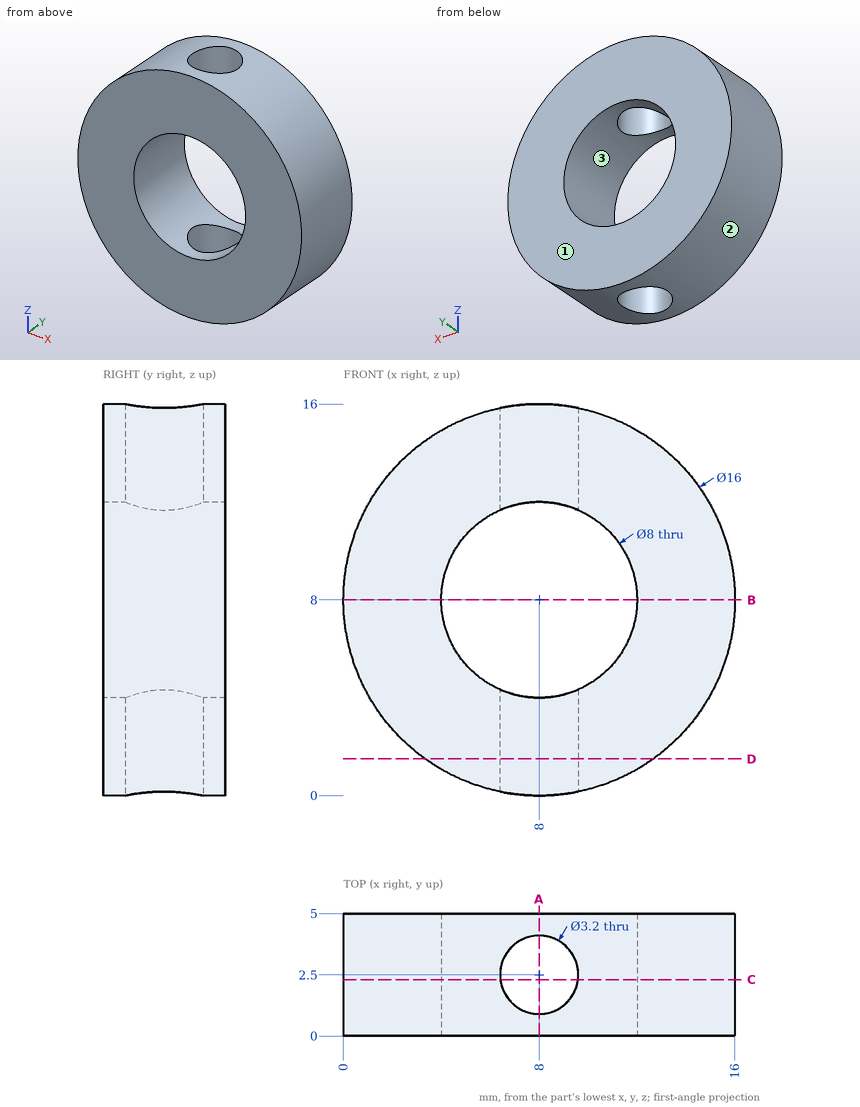
Can you work these out from the drawing? Everything is in mm from the part's minimum corner. Coordinates: 2 decimals unless noted, no trailing zeros. Loops run counter-clockwise (first coordinate to the right, second up) from the corner with the lowest first, then second, coordinate; pieces in that order, holes last. Notation, with made-up numbers: M -30,20.25 L 5,20.25 A6 ccw 5,29.25 Z; hole C 23,-14 d8. An arc over 180 degrees is marked long. Put each result on its own line as item: value. Start each with the question number.
(1) Suppose I cut it at D-D on z = 1.5. Please give me the cut outline in (x, y), then the cut area to 3 significant figures.
(2) Thinking about a two-plate mould opening in Z: for the marked faces 1, 2 and 3, which applies, pulls with the +Z half, pulls with the -Z half, needs draft (parallel to the pull), parting line crosses it, or undercut?
(3) Will this pin go through, and if not, where does the flat tip stop? P1, Ø1, axis at y = 1, z = 5, coming from the -X side.
(4) Suppose I cut it at C-C on y = 2.3. Please give me the cut outline in (x, z).
(5) Suppose I cut it at A-A on x = 8. Please give me the cut outline in (y, z), then the cut area to 3 significant figures.
(6) Suppose I cut it at B-B on z = 8. Please give me the cut outline in (x, y).
(7) I need wall thicknesses on line 1 (X direction, y = 2.35, z = 8.5); line 2 (Z direction, x = 4.5, y = 0.4); line 3 (X direction, y = 3.75, z = 14.5). Which ranges of each line are inside material? Lowest first, please. Write a range as from..to.
Solutions:
1. outline: M 3.34,0 L 12.66,0 L 12.66,5 L 3.34,5 Z; hole C 8,2.5 d3.2
1. area: 38.6 mm2
2. face 1: needs draft
2. face 2: parting line crosses it
2. face 3: undercut
3. P1: stops at x = 0.4
4. outline: M 6.41,0.16 L 6.41,4.33 A4 cw 6.41,11.67 L 6.41,15.84 A8 ccw Z; M 9.59,0.16 A8 ccw 9.59,15.84 L 9.59,11.67 A4 cw 9.59,4.33 Z
5. outline: M 0,0 L 0.9,0 L 0.9,4 L 0,4 Z; M 0,12 L 0.9,12 L 0.9,16 L 0,16 Z; M 4.1,0 L 5,0 L 5,4 L 4.1,4 Z; M 4.1,12 L 5,12 L 5,16 L 4.1,16 Z
5. area: 14.4 mm2
6. outline: M 0,0 L 4,0 L 4,5 L 0,5 Z; M 12,0 L 16,0 L 16,5 L 12,5 Z
7. line 1: x = 0.02..4.03, 11.97..15.98
7. line 2: z = 0.81..6.06, 9.94..15.19
7. line 3: x = 3.34..7, 9..12.66
